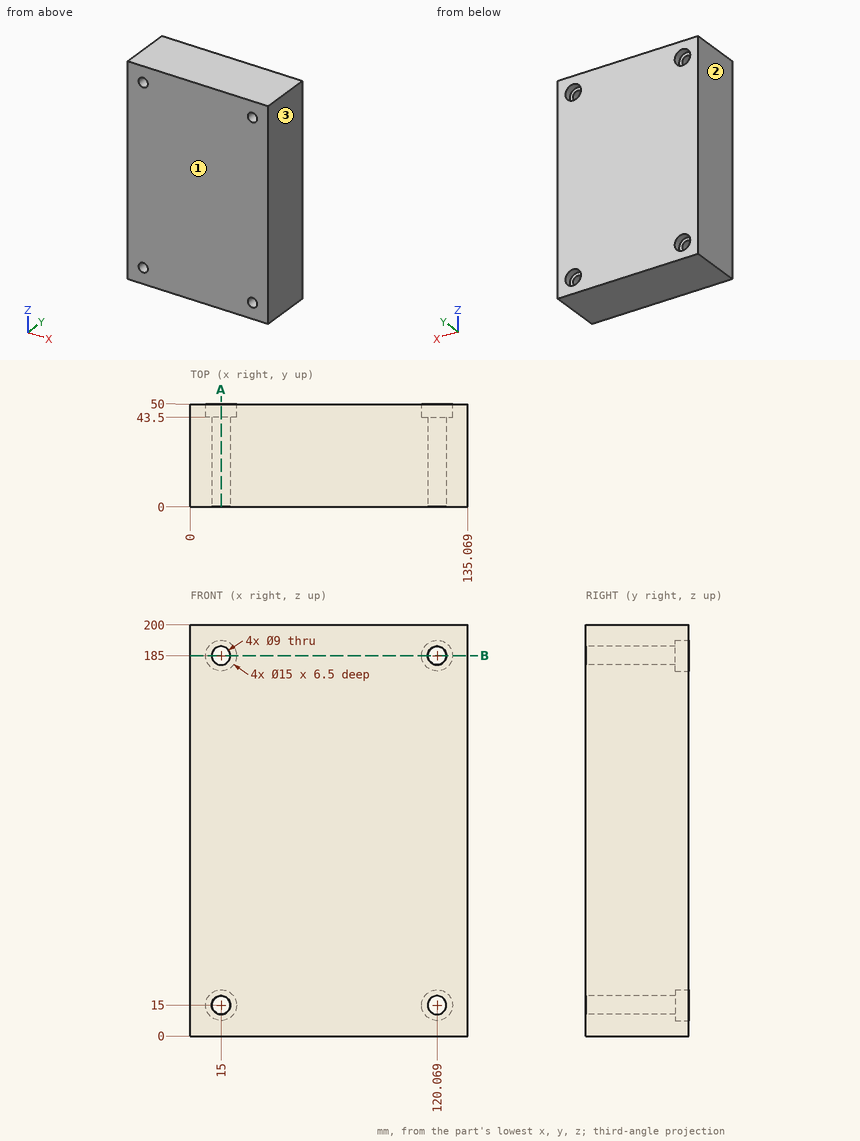
For this review, use the dimensioned drawing (mm, ordinates from the lowest corner) and the shaded views. Coordinates: 2 decimals unless noted, no trailing zeros. Loops run counter-clockwise (first coordinate to the right, second up) from the corner with the lowest first, then second, coordinate; pieces in that order, holes last. Notation, with made-up numbers: (-16, 3.25) -> (6, 3.25) arc R17 ccw to (6, 22.25) -> close; hole circle Ø5 at (32, 54). An arc over 180 degrees is marked (long way). Use a Markdown table: item, result. Add a question column.
Item 1: The part is to be moulded in two halves that separate along X. For the marked faces 1, 2 and 3, say which applies: +X half, -X half, draft (parallel to the pull), parting line (faces both ways), or undercut.
Item 2: We need section A-A, the plane x = 15. Write out the cut boundary in (y, z), and give its area (3 significant figures).
Item 3: Clearance check with a flat-ended pin moving along its axis: P1, Ø7.5, axis at x = 13.5, z = 15.5, coming from the +Y side. State where the tip first meets the part, or that it passes through.
Item 4: Wall thickness on L1, parallel to Z at x = 15, y = 29; L2, parallel to Z at x = 15, y = 47; L3, parallel to X at y = 48, z = 185: over which ranges is each line inside the solid? List them lowest first. Write a range as from..to.
Item 5: We need section B-B, the plane z = 185. Write out the cut boundary in (x, y).
Numbers:
| question | item | result |
|---|---|---|
| 1 | face 1 | draft |
| 1 | face 2 | -X half |
| 1 | face 3 | +X half |
| 2 | outline | (0, 0) -> (50, 0) -> (50, 7.5) -> (43.5, 7.5) -> (43.5, 10.5) -> (0, 10.5) -> close; (0, 19.5) -> (43.5, 19.5) -> (43.5, 22.5) -> (50, 22.5) -> (50, 177.5) -> (43.5, 177.5) -> (43.5, 180.5) -> (0, 180.5) -> close; (0, 189.5) -> (43.5, 189.5) -> (43.5, 192.5) -> (50, 192.5) -> (50, 200) -> (0, 200) -> close |
| 2 | area | 9,020 mm^2 |
| 3 | P1 | stops at y = 43.5 |
| 4 | L1 | z = 0..10.5, 19.5..180.5, 189.5..200 |
| 4 | L2 | z = 0..7.5, 22.5..177.5, 192.5..200 |
| 4 | L3 | x = 0..7.5, 22.5..112.57, 127.57..135.07 |
| 5 | outline | (0, 0) -> (10.5, 0) -> (10.5, 43.5) -> (7.5, 43.5) -> (7.5, 50) -> (0, 50) -> close; (19.5, 0) -> (115.57, 0) -> (115.57, 43.5) -> (112.57, 43.5) -> (112.57, 50) -> (22.5, 50) -> (22.5, 43.5) -> (19.5, 43.5) -> close; (124.57, 0) -> (135.07, 0) -> (135.07, 50) -> (127.57, 50) -> (127.57, 43.5) -> (124.57, 43.5) -> close |
